```python
from build123d import *

# Parameters (mm, degrees)
SKETCH1_W           = 14
SKETCH1_H           = 3
BOSS_EXTRUDE1_DEPTH = 24
CUT_EXTRUDE1_REACH  = 27.179
SKETCH2_R           = 3
SKETCH3_W           = 26
SKETCH3_H           = 3
BOSS_EXTRUDE2_DEPTH = 10
CUT_EXTRUDE2_REACH  = 31.069
FILLET1_R           = 3
FILLET2_R           = 6


with BuildPart() as part:
    # Sketch1 → Boss-Extrude1 (new body)
    with BuildSketch(Plane(origin=(0, 0, 0), x_dir=(1, 0, 0), z_dir=(0, 1, 0))):
        with Locations((0, -1.5)):
            Rectangle(SKETCH1_W, SKETCH1_H)
    extrude(amount=BOSS_EXTRUDE1_DEPTH)

    # Sketch2 → Cut-Extrude1 (cut, up to next)
    with BuildSketch(Plane.XY.offset(3), mode=Mode.PRIVATE) as cut_extrude1_sk1:
        with Locations((0, 6)):
            Circle(SKETCH2_R)
    cut_extrude1_tool1 = extrude(cut_extrude1_sk1.sketch, amount=-CUT_EXTRUDE1_REACH, mode=Mode.PRIVATE) & part.part
    add(cut_extrude1_tool1.solids().sort_by_distance((0, 6, 3))[0], mode=Mode.SUBTRACT)

    # Sketch3 → Boss-Extrude2 (add)
    with BuildSketch(Plane.XY):
        with Locations((0, 22.5)):
            Rectangle(SKETCH3_W, SKETCH3_H)
    extrude(amount=BOSS_EXTRUDE2_DEPTH)

    # Sketch4 → Cut-Extrude2 (cut, up to next)
    with BuildSketch(Plane(origin=(0, 24, 0), x_dir=(1, 0, 0), z_dir=(0, 1, 0)), mode=Mode.PRIVATE) as cut_extrude2_sk1:
        with BuildLine():
            ThreePointArc((8.25, -5.25), (10, -3.5), (11.75, -5.25))
            Line((11.75, -5.25), (11.75, -7.75))
            ThreePointArc((11.75, -7.75), (10, -9.5), (8.25, -7.75))
            Line((8.25, -7.75), (8.25, -5.25))
        make_face()
    cut_extrude2_tool1 = extrude(cut_extrude2_sk1.sketch, amount=-CUT_EXTRUDE2_REACH, mode=Mode.PRIVATE) & part.part
    # Sketch4 → Cut-Extrude2 (cut, up to next)
    with BuildSketch(Plane(origin=(0, 24, 0), x_dir=(1, 0, 0), z_dir=(0, 1, 0)), mode=Mode.PRIVATE) as cut_extrude2_sk2:
        with BuildLine():
            Line((-8.25, -7.75), (-8.25, -5.25))
            ThreePointArc((-8.25, -5.25), (-10, -3.5), (-11.75, -5.25))
            Line((-11.75, -5.25), (-11.75, -7.75))
            ThreePointArc((-11.75, -7.75), (-10, -9.5), (-8.25, -7.75))
        make_face()
    cut_extrude2_tool2 = extrude(cut_extrude2_sk2.sketch, amount=-CUT_EXTRUDE2_REACH, mode=Mode.PRIVATE) & part.part
    add(cut_extrude2_tool1.solids().sort_by_distance((10, 24, 6.5))[0], mode=Mode.SUBTRACT)
    add(cut_extrude2_tool2.solids().sort_by_distance((-10, 24, 6.5))[0], mode=Mode.SUBTRACT)

    # Fillet1
    fillet1_edges = [part.edges().sort_by_distance(p)[0] for p in [
        (13, 22.5, 0),
        (-13, 22.5, 0),
        (13, 22.5, 10),
        (-13, 22.5, 10),
    ]]
    fillet(fillet1_edges, radius=FILLET1_R)

    # Fillet2
    fillet2_edges = [part.edges().sort_by_distance(p)[0] for p in [
        (0, 21, 3),
        (-7, 0, 1.5),
        (7, 0, 1.5),
    ]]
    fillet(fillet2_edges, radius=FILLET2_R)


solid = part.part
```
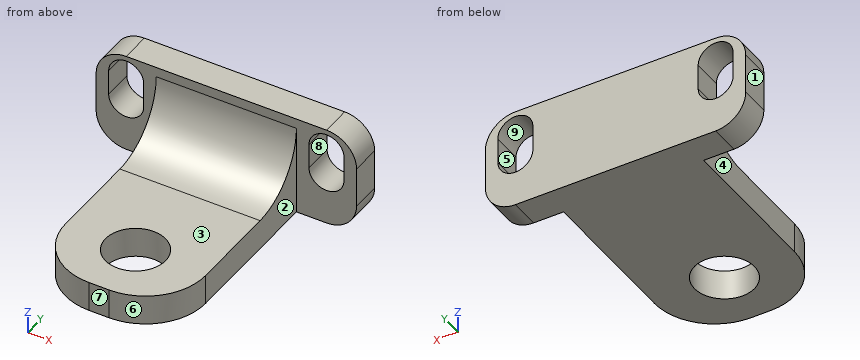
Geometry: final body of the model. Coordinates: model frame, mm. Face numbers are marked on the shaded views. A direction names the side the tool comes from. Round coordinates to 2 decimals unless told otherwise and drop trailing zeros. Order: outer loops, then holes, each group sorted by start corner. A loop starts at its lowest first (then second) coordinate and runs counter-clockwise, first axis right, second up. Notation, with made-up numbers: (9, -12.75) -> (19, -12.75) arc R19 cw to (19, 24.25) -> close; hole circle Ø9 at (-11.75, 61.25). An arc over 180 degrees is marked (long way). Use CSV: the item, a comma, the result in double quotes. Start each with the question number.
1) Set-up query: the marked faces 1, 2, 3, 4 and 5. Return all of +Z, -Z, +X, -X, +Y, -Y with unobstructed straight access to the full face (end or side cutting, diameter ignored); none if empty.
2) Draft query along X for the marked faces 6, 7, 8 and 9. Return one class per face: +X half, -X half, draft (parallel to the pull), parting line (faces both ways), or undercut.
3) Section B-B (x = 1.5). Return the cut outline in (y, z).
4) Material intervals for line 1 along X through (y, z) = (22.5, 8.25); line 2 along Y through (x, z) = (0, 2); line 3 along Y through (x, z) = (8.5, 3.75), sorted ascending. Write a range as from..to.
5) Section A-A (z = 8.5). State how many separate pieces and enclosed holes the cut face has, and give its area (3 significant figures).
6) First-contact query: pin 1 Ø4 at (x, y) = (0, 10) entering from +Z; pin 2 Ø5 at (x, z) = (-3, 6) entering from -Y; pin 3 Ø3 at (y, z) = (4, 1.5) entering from +X; pin 4 Ø2.5 at (y, z) = (16, 4.5) entering from +X. Flat tips, straight axial feed; report the tip coordinate or a pass-through.
7) Section D-D (z = 1.5). Return the cut outline in (x, y).
8) Section C-C (y = 4). Return the cut outline in (x, z), and give its area (3 significant figures).
Returned:
1,face 1,"+Z, -Z, -X, +Y, -Y"
1,face 2,"+Z, -Z, +X, -Y"
1,face 3,"+Z, +X, -X, -Y"
1,face 4,"+Z, -Z, -X, -Y"
1,face 5,"+Y, -Y"
2,face 6,"+X half"
2,face 7,"draft"
2,face 8,"undercut"
2,face 9,"undercut"
3,outline,"(0.02, 0) -> (3.4, 0) -> (3.4, 3) -> (0.02, 3) -> close; (8.6, 0) -> (24, 0) -> (24, 10) -> (21, 10) -> (21, 9) arc R6 cw to (15, 3) -> (8.6, 3) -> close"
4,line 1,"x = -12.73..-11.68, -8.32..8.32, 11.68..12.73"
4,line 2,"y = 0..3, 9..24"
4,line 3,"y = 21..24"
5,separate pieces,"3"
5,enclosed holes,"0"
5,area,"56.9 mm²"
6,pin 1,"stops at z = 3"
6,pin 2,"stops at y = 17.4"
6,pin 3,"stops at x = 6.98"
6,pin 4,"passes through"
7,outline,"(-12.6, 21) -> (-7, 21) -> (-7, 6) arc R6 ccw to (-1, 0) -> (1, 0) arc R6 ccw to (7, 6) -> (7, 21) -> (12.6, 21) -> (12.6, 24) -> (-12.6, 24) -> close; hole circle Ø6 at (0, 6)"
8,outline,"(-6.66, 0) -> (-2.24, 0) -> (-2.24, 3) -> (-6.66, 3) -> close; (2.24, 0) -> (6.66, 0) -> (6.66, 3) -> (2.24, 3) -> close"
8,area,"26.5 mm²"
